Here's how the part is built. I have some questions about the finished solid (model axes, mm). Coordinates: 2 decimals unless noted, no trailing zeros. Write each loop counter-clockwise with the first axis right and the second up, starting at its lowest first coordinate (ties: lowest second). Pieces come first, ordered by that corner, then holes. Notation, with made-up numbers: (-6, 88) -> (20, 88) arc R3 cw to (20, 92) -> close; hole circle Ø11 at (44.5, -32.5). An arc over 180 degrees is marked (long way). Use a Markdown table: item, result. Add a question column.
Autodesk Inventor part; units mm, degrees
ref_plane "YZ Plane" through (0, 0, 0) normal (1, 0, 0) x (0, 1, 0)
ref_plane "XZ Plane" through (0, 0, 0) normal (0, 1, 0) x (-1, 0, 0)
ref_plane "XY Plane" through (0, 0, 0) normal (0, 0, 1) x (1, 0, 0)
sketch "Skizze1" plane through (0, 0, 0) normal (0, 0, 1) x (1, 0, 0)
  circle A0 centre (0, 0) radius 25
  line L0 (-32.5, 32.5) -> (32.5, 32.5)
  line L1 (32.5, 22.5) -> (32.5, -22.5)
  line L2 (22.5, -32.5) -> (-22.5, -32.5)
  line L3 (-32.5, -22.5) -> (-32.5, 22.5)
  line L4 (-32.5, 32.5) -> (32.5, -32.5) construction
  line L5 (32.5, 32.5) -> (-32.5, -32.5) construction
  circle A1 centre (-25, 25) radius 1.9
  circle A2 centre (25, 25) radius 1.9
  circle A3 centre (-25, -25) radius 1.9
  circle A4 centre (25, -25) radius 1.9
  line L6 (-22.5, 32.5) -> (22.5, 32.5)
  line L7 (32.5, -32.5) -> (-32.5, -32.5)
  line L8 (-32.5, -32.5) -> (-32.5, 32.5)
  line L9 (32.5, 32.5) -> (32.5, -32.5)
  arc A5 (-22.5, 32.5) -> (-32.5, 22.5) centre (-22.5, 22.5) ccw
  arc A6 (-32.5, -22.5) -> (-22.5, -32.5) centre (-22.5, -22.5) ccw
  arc A7 (22.5, -32.5) -> (32.5, -22.5) centre (22.5, -22.5) ccw
  arc A8 (32.5, 22.5) -> (22.5, 32.5) centre (22.5, 22.5) ccw
  dimension "d0" = 50
  dimension "d1" = 65
  dimension "d2" = 65
  dimension "d5" = 25
  dimension "d6" = 25
  dimension "d7" = 3.8
  dimension "d10" = 50
  dimension "d13" = 50
  dimension "d16" = 10
extrude "Extrusion1" add sketch "Skizze1" along normal blind 6 contours L0 A8 L1 A7 L2 A6 L3 A5
chamfer "Fase1" distance 0.5 angle 45 16 edges at (29.5711, 29.5711, 0) (0, 32.5, 0) (-29.5711, 29.5711, 0) (-32.5, 0, 0) (-29.5711, -29.5711, 0) (0, -32.5, 0) (29.5711, -29.5711, 0) (32.5, 0, 0) (29.5711, 29.5711, 6) (0, 32.5, 6) (-29.5711, 29.5711, 6) (-32.5, 0, 6) (-29.5711, -29.5711, 6) (0, -32.5, 6) (29.5711, -29.5711, 6) (32.5, 0, 6)
properties part number "StageInsert_FoilHolder_Part2"
Q1. Suppose I cut it at A-A, the plane x = 0. Write out the boundary of the cut face in (y, z), and give its area (3 significant figures).
Q2. Suppose I cut it at C-C, the plane z = 2.5. Write out the boundary of the cut face in (x, y), and give its area (3 significant figures).
Q3. Please list where these lines run through material, in increasing order: line 1 (X direction, y = -14, z = 2.3); line 2 (X direction, y = 22.5, z = 4.8); line 3 (Y direction, x = 0, z = 0.9).
Q4. Will these pins go through, and if not, where does the flat tip stop? pin 1 (1 mm diameter, centred on x = -21, y = 11, fed in from -Z); pin 2 (1.5 mm diameter, centred on x = -26, z = 4.5, fed in from +Y).
Q5. Thinking about a two-plate mould opening in X: for faces 1 (the conical face through (29.39, -29.24, 5.86)), 2 (the cylindrical face through (23.846, -7.509, 2.958)), 3 (the cylindrical face through (-25.247, -26.884, 2.958)), 4 (the cylindrical face through (-29.65, 29.49, 2.96)), which applies, released by +X, released by -X, zero draft, split by the parting line, or undercut?
Answer key:
| question | item | result |
|---|---|---|
| 1 | outline | (-32.5, 0.5) -> (-32, 0) -> (-25, 0) -> (-25, 6) -> (-32, 6) -> (-32.5, 5.5) -> close; (25, 0) -> (32, 0) -> (32.5, 0.5) -> (32.5, 5.5) -> (32, 6) -> (25, 6) -> close |
| 1 | area | 89.5 mm^2 |
| 2 | outline | (-32.5, -22.5) arc R10 ccw to (-22.5, -32.5) -> (22.5, -32.5) arc R10 ccw to (32.5, -22.5) -> (32.5, 22.5) arc R10 ccw to (22.5, 32.5) -> (-22.5, 32.5) arc R10 ccw to (-32.5, 22.5) -> close; hole circle Ø3.8 at (-25, -25); hole circle Ø3.8 at (-25, 25); hole circle Ø50 at (0, 0); hole circle Ø3.8 at (25, -25); hole circle Ø3.8 at (25, 25) |
| 2 | area | 2,130 mm^2 |
| 3 | line 1 | x = -32.5 to -20.71, 20.71 to 32.5 |
| 3 | line 2 | x = -32.5 to -10.9, 10.9 to 32.5 |
| 3 | line 3 | y = -32.5 to -25, 25 to 32.5 |
| 4 | pin 1 | passes through |
| 4 | pin 2 | stops at y = 32.11 |
| 5 | face 1 | released by +X |
| 5 | face 2 | undercut |
| 5 | face 3 | undercut |
| 5 | face 4 | released by -X |
